The listing builds one solid part. Answer for the finished solid, in the listing's coordinates (mm). Face numbers are marked on the shaded views. A direction names the side the tool comes from. Round coordinates to 2 decimals unless told otherwise and drop trailing zeros. Write each loop counter-clockwise with the first axis right and the second up, starting at its lowest first coordinate (ties: lowest second). Pieces come first, ordered by that corner, then holes. Notation, with made-up numbers: (-3, 81) - (49, 81) arc R11 cw to (49, 95) - close; hole circle Ø8 at (-7, -37.75). An arc over 180 degrees is marked (long way). Return JSON: item names as keys, results as strings. Group by question number.
(1) Find the intervals of material crossed by line 1 along X through (y, z) = (-24, 0.25); line 2 along X through (y, z) = (-2, 2.45); line 3 along Y through (x, z) = (-8.5, 3.6), in increasing order. Write a range as [from, to].
(2) Section C-C, the plane y = -26.5 is taken. Write down the section's boundary in (x, z), then the cut area to 3 significant figures.
(3) Which of the six approach directions +Z, -Z, +X, -X, +Y, -Y give full straight-line access (tool end or side, diameter ignored) to the marked faces 1, 2, 3 and 4?
(4) Each of these flat-tipped pins is pushed along its axis until it touches: pin 1 (2 mm diameter, centred on x = -39.5, z = 3, fed in from -Y); pin 2 (5 mm diameter, centred on x = -19, y = -4, fed in from -Z); pin 3 (2 mm diameter, centred on x = -39.5, z = 1.5, fed in from +Y); pin 4 (1.9 mm diameter, centred on x = -10, y = -15.5, fed in from -Z). Where does it stop, or does it pass through?
(5) Section A-A, the plane z = 0.8 is taken. Write down the section's boundary in (x, y).
(6) Section B-B, the plane y = -15.5 is taken. Write down the section's boundary in (x, z), then the cut area to 3 significant figures.
```python
from build123d import *

# Parameters (mm, degrees)
SALIENTE_EXTRUIR1_DEPTH = 4
CORTAR_EXTRUIR1_REACH   = 55.16
CROQUIS2_R              = 1.04775


with BuildPart() as part:
    # Croquis1 → Saliente-Extruir1 (new body)
    with BuildSketch(Plane.XY):
        Polygon((-35, 0), (-35, -4), (-43, -4), (-43, -27), (-35, -27), (-35, -31), (-10, -31), (-10, -27), (-8, -27), (-8, -22), (-5, -22), (-5, -9), (-8, -9), (-8, -4), (-10, -4), (-10, 0), align=None)
    extrude(amount=SALIENTE_EXTRUIR1_DEPTH)

    # Croquis2 → Cortar-Extruir1 (cut, up to next)
    with BuildSketch(Plane.XY.offset(4), mode=Mode.PRIVATE) as cortar_extruir1_sk1:
        with Locations((-38.00175, -15.5)):
            Circle(CROQUIS2_R)
    cortar_extruir1_tool1 = extrude(cortar_extruir1_sk1.sketch, amount=-CORTAR_EXTRUIR1_REACH, mode=Mode.PRIVATE) & part.part
    # Croquis2 → Cortar-Extruir1 (cut, up to next)
    with BuildSketch(Plane.XY.offset(4), mode=Mode.PRIVATE) as cortar_extruir1_sk2:
        with Locations((-9.99825, -15.5)):
            Circle(CROQUIS2_R)
    cortar_extruir1_tool2 = extrude(cortar_extruir1_sk2.sketch, amount=-CORTAR_EXTRUIR1_REACH, mode=Mode.PRIVATE) & part.part
    add(cortar_extruir1_tool1.solids().sort_by_distance((-38.00175, -15.5, 4))[0], mode=Mode.SUBTRACT)
    add(cortar_extruir1_tool2.solids().sort_by_distance((-9.99825, -15.5, 4))[0], mode=Mode.SUBTRACT)


solid = part.part
```
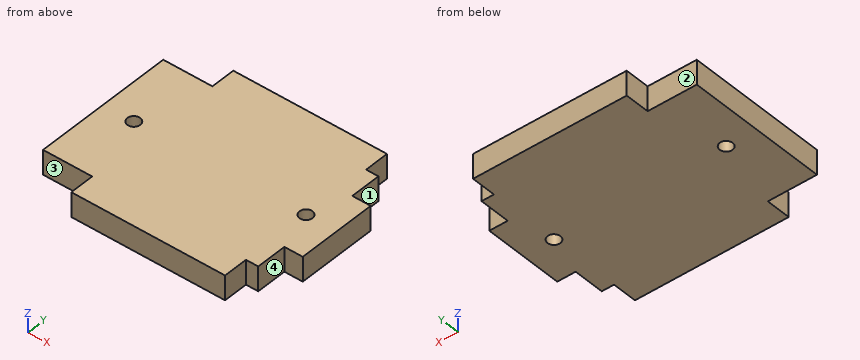
Working result:
{
 "1": {"line 1": "x = [-43, -8]", "line 2": "x = [-35, -10]", "line 3": "y = [-27, -4]"},
 "2": {"outline": "(-43, 0) - (-8, 0) - (-8, 4) - (-43, 4) - close", "area": "140 mm^2"},
 "3": {"face 1": "+Z, -Z, +X, +Y", "face 2": "+Z, -Z, -X, +Y", "face 3": "+Z, -Z, -X, -Y", "face 4": "+Z, -Z, +X, -Y"},
 "4": {"pin 1": "stops at y = -27", "pin 2": "stops at z = 0", "pin 3": "stops at y = -4", "pin 4": "passes through"},
 "5": {"outline": "(-43, -27) - (-35, -27) - (-35, -31) - (-10, -31) - (-10, -27) - (-8, -27) - (-8, -22) - (-5, -22) - (-5, -9) - (-8, -9) - (-8, -4) - (-10, -4) - (-10, 0) - (-35, 0) - (-35, -4) - (-43, -4) - close; hole circle Ø2.1 at (-38, -15.5); hole circle Ø2.1 at (-10, -15.5)"},
 "6": {"outline": "(-43, 0) - (-39.05, 0) - (-39.05, 4) - (-43, 4) - close; (-36.95, 0) - (-11.05, 0) - (-11.05, 4) - (-36.95, 4) - close; (-8.95, 0) - (-5, 0) - (-5, 4) - (-8.95, 4) - close", "area": "135 mm^2"}
}
